The figure shows three views and two pictorial views of one solid part (mm, origin at its lowest corner). Answer the questions. Give positions to 0.01 mm unless a question says otherwise; leave off trailing zeros. Write each loop counter-clockwise with the first axis right and the second up, starting at its lowest first coordinate (ties: lowest second). Pieces come first, ordered by that corner, then holes. Notation, with made-up numbers: (38, 48.25) -> (62, 48.25) arc R10 ccw to (62, 59.25) -> close; hole circle Ø1 at (-28, -30.5). An arc over 180 degrees is marked (long way). Use a Markdown table: item, result.
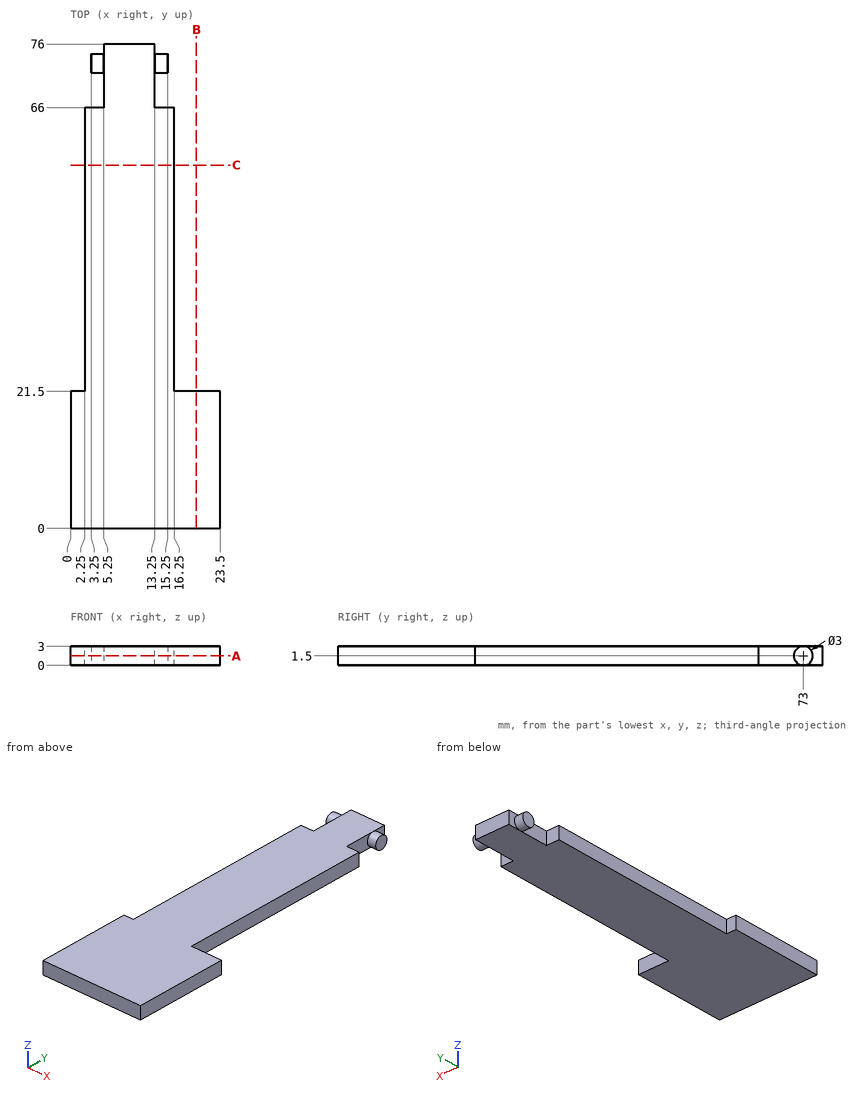
Item 1: Each of these flat-tipped pins is pushed along its axis until it touches: P1, Ø1.5, axis at y = 60.5, z = 1.5, coming from the +X side; P2, Ø3, axis at x = 6, y = 64, coming from the -Z side; P3, Ø0.9, axis at y = 36.5, z = 2, coming from the -X side; P4, Ø0.9, axis at y = 68, z = 1.5, coming from the -X side. Where does it stop, or does it pass through?
Return value:
| item | result |
|---|---|
| P1 | x = 16.25 |
| P2 | z = 0 |
| P3 | x = 2.25 |
| P4 | x = 5.25 |
Item 2: A cutting plane is placed at B-B (x = 19.75). Give the vertices of the cut face in (y, z).
Return value:
| item | result |
|---|---|
| outline | (0, 0) -> (21.5, 0) -> (21.5, 3) -> (0, 3) -> close |
Item 3: A cutting plane is placed at C-C (y = 57). Give the vertices of the cut face in (x, z).
Return value:
| item | result |
|---|---|
| outline | (2.25, 0) -> (16.25, 0) -> (16.25, 3) -> (2.25, 3) -> close |
Item 4: Straight lines are drawn through the part: line 1 along X through (y, z) = (27, 1.85); line 2 along Y through (x, z) = (16, 0.2); line 3 along Y through (x, z) = (17, 0.7). For each, find the intervals that lie inside material, in ascending order. Write a range as [from, to].
Return value:
| item | result |
|---|---|
| line 1 | [2.25, 16.25] |
| line 2 | [0, 66] |
| line 3 | [0, 21.5] |
Item 5: A cutting plane is placed at A-A (z = 1.5). Give the vertices of the cut face in (x, y).
Return value:
| item | result |
|---|---|
| outline | (0, 0) -> (23.5, 0) -> (23.5, 21.5) -> (16.25, 21.5) -> (16.25, 66) -> (13.25, 66) -> (13.25, 71.5) -> (15.25, 71.5) -> (15.25, 74.5) -> (13.25, 74.5) -> (13.25, 76) -> (5.25, 76) -> (5.25, 74.5) -> (3.25, 74.5) -> (3.25, 71.5) -> (5.25, 71.5) -> (5.25, 66) -> (2.25, 66) -> (2.25, 21.5) -> (0, 21.5) -> close |
